Input: dimensioned drawing with shaded views. Units: mm. Origin: part minimum x, y, z. A direction names the side the tool comes from. Coordinates: 2 decimals unless noted, no trailing zeros. Loops run counter-clockwise (first coordinate to the right, second up) from the corner with the lowest first, then second, coordinate; pieces in that order, holes last.
Item 1: Section query B-B, the plane z = 3.5. Return the cut outline in (x, y).
Item 2: Pin query (flat end, axial travel): pin 1 Ø2.5 at (y, z) = (10, 3.5) entering from +X; pin 2 Ø8 at (y, z) = (12.5, 18.5) entering from -X; pin 3 Ø4 at (x, z) = (7, 22.5) entering from +Y; pin 4 Ø6 at (x, z) = (14, 15) entering from -Y. Return the tip coordinate at first contact, or that it passes through.
Item 3: Reachability of the marked faces 3 and 4 from +Z, -Z, +X, -X, +Y, -Y: full face, straight path, thin tool, end or side. Return the list, or none.
Item 4: Section query A-A, the plane y = 10. Return the cut outline in (x, z).
Item 5: Pull-direction query (Y, two-part tool) for the marked faces 1 and 2; classes: +Y half, -Y half, draft (parallel to the pull), parting line (faces both ways), or undercut.
Item 6: Section query C-C, the plane x = 10. Return the cut outline in (y, z), then the cut area to 3 significant figures.
Item 7: Section query D-D, the plane z = 17. Return the cut outline in (x, y), then the cut area to 3 significant figures.
Item 8: Line query: probe 1 along Y at (x, z) = (10.1, 3.5); probe 2 along Y at (x, z) = (11.3, 3.5); probe 3 along Z at (x, y) = (2, 12.5). Output: solid intervals per line, ascending.
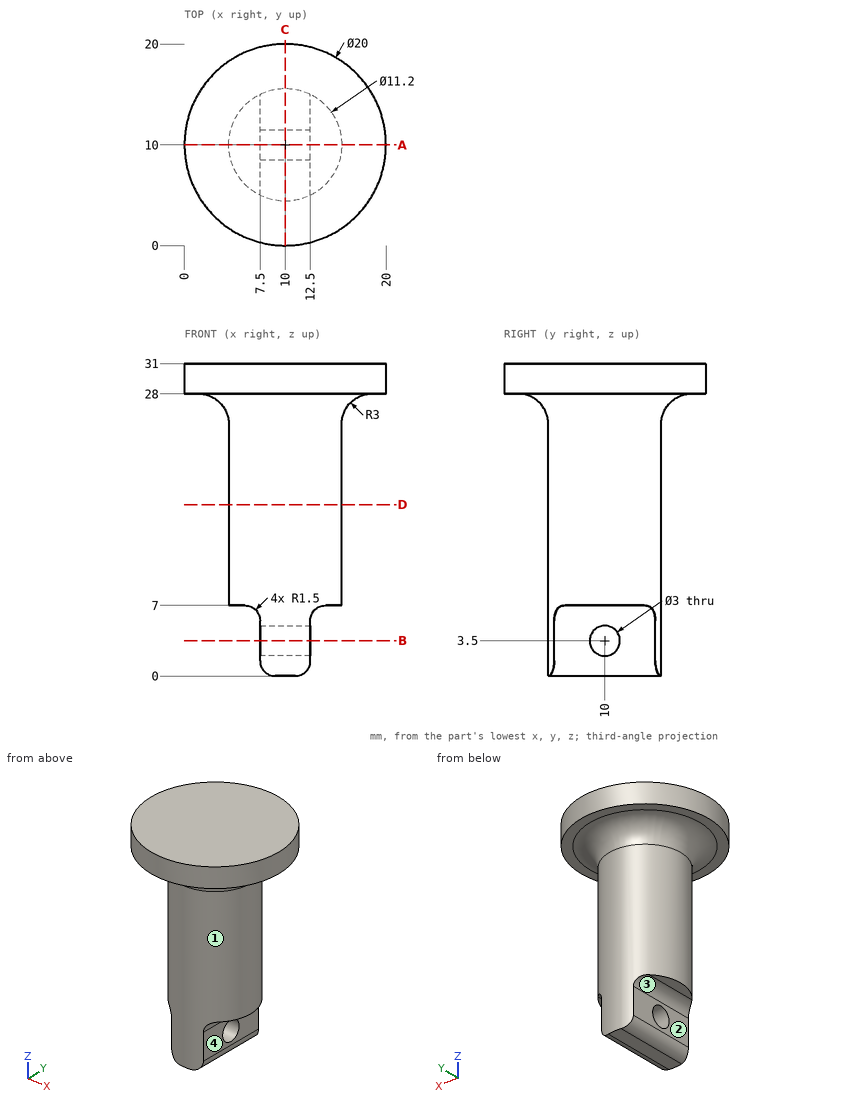
Verdict:
1. outline: (7.5, 4.99) arc R5.6 ccw to (12.5, 4.99) - (12.5, 8.5) - (7.5, 8.5) - close; (7.5, 11.5) - (12.5, 11.5) - (12.5, 15.01) arc R5.6 ccw to (7.5, 15.01) - close
2. pin 1: passes through
2. pin 2: stops at x = 4.4
2. pin 3: stops at y = 15.51
2. pin 4: stops at y = 4.49
3. face 3: -Z, -X, +Y, -Y
3. face 4: -Z, +X, +Y, -Y
4. outline: (0, 28) - (1.4, 28) arc R3 cw to (4.4, 25) - (4.4, 7) - (6, 7) arc R1.5 cw to (7.5, 5.5) - (7.5, 5) - (12.5, 5) - (12.5, 5.5) arc R1.5 cw to (14, 7) - (15.6, 7) - (15.6, 25) arc R3 cw to (18.6, 28) - (20, 28) - (20, 31) - (0, 31) - close; (7.5, 1.5) arc R1.5 ccw to (9, 0) - (11, 0) arc R1.5 ccw to (12.5, 1.5) - (12.5, 2) - (7.5, 2) - close
5. face 1: parting line
5. face 2: draft
6. outline: (0, 28) - (1.4, 28) arc R3 cw to (4.4, 25) - (4.4, 0) - (15.6, 0) - (15.6, 25) arc R3 cw to (18.6, 28) - (20, 28) - (20, 31) - (0, 31) - close; hole circle Ø3 at (10, 3.5)
6. area: 370 mm2
7. outline: circle Ø11.2 at (10, 10)
7. area: 98.5 mm2
8. probe 1: y = 4.4 to 8.5, 11.5 to 15.6
8. probe 2: y = 4.55 to 8.5, 11.5 to 15.45
8. probe 3: z = 27.99 to 31
